Answer from the drawing. Dimensions are ordinates in mm from the lowest x, y and z of the part. Round coordinates to 2 decimals unless told otherwise and drop trailing zeros. Order: outer loops, then holes, each group sorted by start corner. A loop starts at its lowest first (then second) coordinate and runs counter-clockwise, first axis right, second up. Notation, with made-up numbers: (-24, 74.25) -> (-6, 74.25) arc R18 cw to (-6, 97.25) -> close; hole circle Ø2 at (-9.75, 64). An arc over 180 degrees is marked (long way). Use a Markdown table: item, result. Add a question column.
1. Section C-C, the plane y = 71 is taken. Give the vertices of the cut face in (x, z), then the cut area to 3 significant figures.
2. Consider L1, parallel to X at y = 7, z = 4.25; L2, parallel to X at y = 66.5, z = 4.5 (3 decimals); L3, parallel to Y at x = 37, z = 4. Determine where each line is inside the solid, lowest interval first. Write a range as [from, to].
3. Given pin 1 (1.5 mm diameter, centred on x = 47, z = 4, fed in from +Y); pin 2 (2 mm diameter, centred on y = 58, z = 1.5, fed in from +X); pin 3 (10 mm diameter, centred on x = 25.5, y = 69, fed in from -Z); pin 4 (3 mm diameter, centred on x = 31.5, z = 7, fed in from +Y), each flat-ended and moving along its own axis, determine where each tip first touches the part or whether it passes through.
4. Section B-B, the plane x = 5 is taken. Give the vertices of the cut face in (y, z), then the cut area to 3 significant figures.
5. Section A-A, the plane z = 1.25 is taken. Give the vertices of the cut face in (x, y).
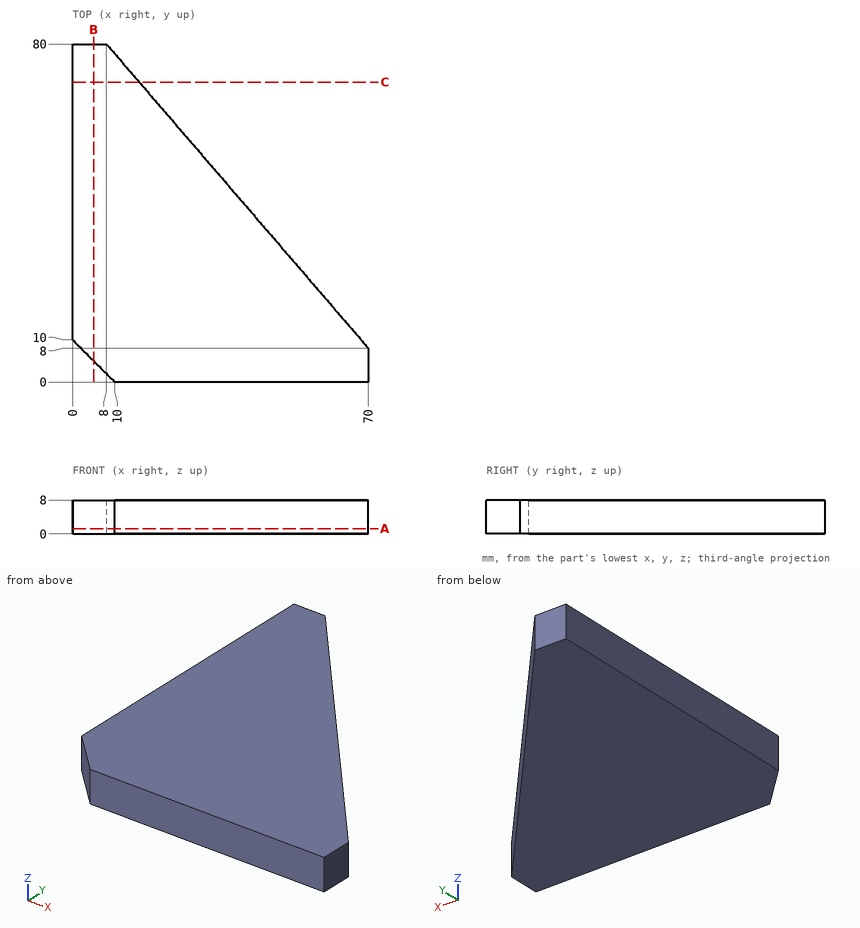
Verdict:
| question | item | result |
|---|---|---|
| 1 | outline | (0, 0) -> (15.75, 0) -> (15.75, 8) -> (0, 8) -> close |
| 1 | area | 126 mm2 |
| 2 | L1 | x = [3, 70] |
| 2 | L2 | x = [0, 19.625] |
| 2 | L3 | y = [0, 46.32] |
| 3 | pin 1 | stops at y = 35.58 |
| 3 | pin 2 | stops at x = 27.81 |
| 3 | pin 3 | passes through |
| 3 | pin 4 | stops at y = 54.45 |
| 4 | outline | (5, 0) -> (80, 0) -> (80, 8) -> (5, 8) -> close |
| 4 | area | 600 mm2 |
| 5 | outline | (0, 10) -> (10, 0) -> (70, 0) -> (70, 8) -> (8, 80) -> (0, 80) -> close |
